Model file for the job. Use its own axes, mm. Face numbers are marked on the shaded views. A direction names the side the tool comes from. Coordinates: 2 decimals unless noted, no trailing zeros. Write each loop counter-clockwise with the first axis right and the second up, starting at its lowest first coordinate (ties: lowest second). Pieces come first, ordered by that corner, then holes.
Q1. Band-saw the part on A-A, the plane z = 54. Write the cut outline in (x, y), plus the area to 3 significant figures.
Q2. Band-saw the part on B-B, the plane x = 49.25. Write the cut outline in (y, z).
Q3. Drill centre lines: probe 1 along Y at (x, z) = (51, 15); probe 2 along Z at (x, y) = (51.25, 21.5); probe 3 along X at (y, z) = (2.5, 63.5). Where is each one in solid material? Low to high.
Q4. Band-saw the part on D-D, the plane y = 11. Write the cut outline in (x, z), plus the area to 3 significant figures.
Q5. Band-saw the part on C-C, the plane z = 4. Write the cut outline in (x, y), plus the area to 3 significant figures.
Q6. Pull direction Z, two halves, no side cores. Call the marked faces 4, 5, 6 and 7: released by +Z, released by -Z, zero draft, split by the parting line, or undercut.
Q7. Which spindle directions (+Z, -Z, +X, -X, +Y, -Y) get a long thin tool onto all of the face, cutting with end or side? Do the marked faces 1, 2 and 3. Say none if no direction does.
Q8. Pin check, flat tips, straight feed: P1, Ø9.5, axis at y = 21.5, z = 15, coming from the +X side; P2, Ø9.5, axis at x = 51, y = 6, coming from the +Z side; P3, Ø2.5, axis at x = 61, z = 40.5, coming from the +Y side. Stop position of each tip, or through.
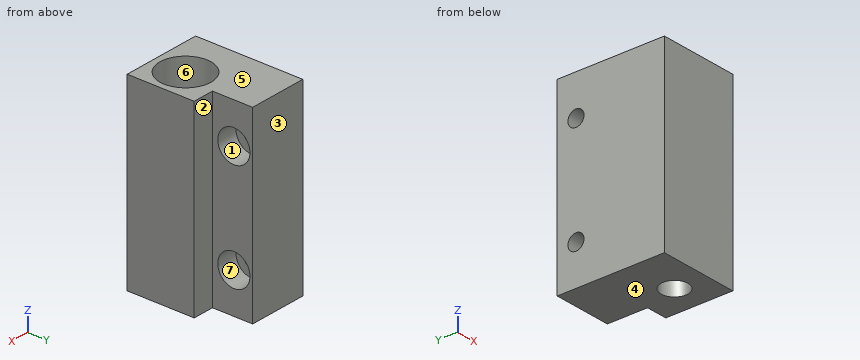
from build123d import *

# Parameters (mm, degrees)
SKETCH_1_W          = 30
SKETCH_1_H          = 40
EXTRUDE_1_DEPTH     = 70
SKETCH_3_R          = 3
CUT_EXTRUDE_1_DEPTH = 70
SKETCH_4_R          = 6
CUT_EXTRUDE_2_DEPTH = 16
SKETCH_5_W          = 8
SKETCH_5_H          = 15
CUT_EXTRUDE_3_DEPTH = 75
SKETCH_2_R          = 9.5
CUT_EXTRUDE_4_DEPTH = 60
SKETCH_6_R          = 5
CUT_EXTRUDE_5_DEPTH = 50


with BuildPart() as part:
    # 草图1 → 凸台-拉伸1 (new body)
    with BuildSketch(Plane.XY):
        with Locations((47.847642857, 10.842857143)):
            Rectangle(SKETCH_1_W, SKETCH_1_H)
    extrude(amount=EXTRUDE_1_DEPTH)

    # 草图3 → 切除-拉伸1 (cut)
    with BuildSketch(Plane(origin=(62.847642857, 0, 0), x_dir=(0, 0, -1), z_dir=(1, 0, 0))):
        with Locations((-55, 23.842857143)):
            Circle(SKETCH_3_R)
        with Locations((-15, 23.842857143)):
            Circle(SKETCH_3_R)
    extrude(amount=-CUT_EXTRUDE_1_DEPTH, mode=Mode.SUBTRACT)

    # 草图4 → 切除-拉伸2 (cut)
    with BuildSketch(Plane(origin=(62.847642857, 0, 0), x_dir=(0, 0, -1), z_dir=(1, 0, 0))):
        with Locations((-55, 23.842857143)):
            Circle(SKETCH_4_R)
        with Locations((-15, 23.842857143)):
            Circle(SKETCH_4_R)
    extrude(amount=-CUT_EXTRUDE_2_DEPTH, mode=Mode.SUBTRACT)

    # 草图5 → 切除-拉伸3 (cut)
    with BuildSketch(Plane.XY.offset(70)):
        with Locations((58.847642857, 23.342857143)):
            Rectangle(SKETCH_5_W, SKETCH_5_H)
    extrude(amount=-CUT_EXTRUDE_3_DEPTH, mode=Mode.SUBTRACT)

    # 草图2 → 切除-拉伸4 (cut)
    with BuildSketch(Plane.XY.offset(70)):
        with Locations((51.107196317, 2.608195772)):
            Circle(SKETCH_2_R)
    extrude(amount=-CUT_EXTRUDE_4_DEPTH, mode=Mode.SUBTRACT)

    # 草图6 → 切除-拉伸5 (cut)
    with BuildSketch(Plane.XY.offset(10)):
        with Locations((51.107196317, 2.608195772)):
            Circle(SKETCH_6_R)
    extrude(amount=-CUT_EXTRUDE_5_DEPTH, mode=Mode.SUBTRACT)


solid = part.part
Answer sheet:
1. outline: (32.85, -9.16) - (62.85, -9.16) - (62.85, 15.84) - (54.85, 15.84) - (54.85, 17.93) - (46.85, 17.93) - (46.85, 21.01) - (32.85, 21.01) - close; (32.85, 26.67) - (46.85, 26.67) - (46.85, 29.76) - (54.85, 29.76) - (54.85, 30.84) - (32.85, 30.84) - close; hole circle Ø19 at (51.11, 2.61)
1. area: 623 mm2
2. outline: (-9.16, 0) - (-2.03, 0) - (-2.03, 10) - (-6.71, 10) - (-6.71, 70) - (-9.16, 70) - close; (7.25, 0) - (30.84, 0) - (30.84, 70) - (11.92, 70) - (11.92, 10) - (7.25, 10) - close; hole circle Ø12 at (23.84, 15); hole circle Ø12 at (23.84, 55)
3. probe 1: y = -9.16 to -6.89, 12.11 to 17.84, 29.84 to 30.84
3. probe 2: z = 0 to 9.48, 20.52 to 49.48, 60.52 to 70
3. probe 3: x = 32.85 to 41.61, 60.61 to 62.85
4. outline: (32.85, 0) - (62.85, 0) - (62.85, 70) - (55.56, 70) - (55.56, 10) - (46.65, 10) - (46.65, 70) - (32.85, 70) - close
4. area: 1,570 mm2
5. outline: (32.85, -9.16) - (62.85, -9.16) - (62.85, 15.84) - (54.85, 15.84) - (54.85, 30.84) - (32.85, 30.84) - close; hole circle Ø10 at (51.11, 2.61)
5. area: 1,000 mm2
6. face 4: released by -Z
6. face 5: released by +Z
6. face 6: zero draft
6. face 7: undercut
7. face 1: +X
7. face 2: +Z, -Z, +X, +Y
7. face 3: +Z, -Z, +X, -X, +Y
8. P1: stops at x = 54.85
8. P2: stops at z = 10
8. P3: stops at y = 15.84
